Geometry: final body of the model. Coordinates: model frame, mm. A direction names the side the tool comes from. Round coordinates to 2 decimals unless told otherwise and drop trailing zeros. Loops run counter-clockwise (first coordinate to the right, second up) from the corner with the lowest first, then second, coordinate; pieces in that order, holes last. Notation, with made-up numbers: (18.25, 8.5) - (71.25, 8.5) arc R23 cw to (71.25, 47.5) - close; hole circle Ø1 at (-13, 6). An arc over 180 degrees is marked (long way). Write item = value, one per line. Start each with the question number.
Item 1: Section A-A (z = -12). Return loops of the section in (x, y).
Item 2: First-contact query: pin 1 (1 mm diameter, centred on x = 3.5, y = 3.5, fed in from +Z); pin 2 (4 mm diameter, centred on x = 0.5, y = -0.5, fed in from +Z); pin 3 (4 mm diameter, centred on y = 2.5, z = -5.5, fed in from -X). Flat tips, straight axial feed; report the tip coordinate or a pass-through.
Item 3: Line query: line 1 (Y direction, x = 0, z = -11.75); line 2 (Y direction, x = -3.5, z = -3.25). Output: solid intervals per line, ascending. Write a range as from..to.
Item 4: Draft query along Y for faces 3 (the conical face through (-2.24, 0.71, 5.54)), 4 (the cylindrical face through (-5.96, 1.88, -7.43)). Return one class per face: pulls with the +Y half, pulls with the -Y half, needs draft (parallel to the pull), parting line crosses it, or undercut.
Item 5: Access query for faces 1 (the cylindrical face through (-2.285, 3.584, -7.155)), 2 (the conical face through (-1.74, -3.345, 6.363)). Directions: +Z, -Z, +X, -X, +Y, -Y. A direction counts if a zero-diameter tool reaches every point of the face in a straight line with its end or side. Return the directions, or none.
from build123d import *

# Parameters (mm, degrees)
F2_R = 0.8


with BuildPart() as f1:
    # F0 (on Front) → F1 (revolve)
    with BuildSketch(Plane.XZ):
        Polygon((-4.25, 2.833334), (-1.375272, 6.924292), (-3.375272, 6.924292), (-6.25, 2.833334), (-6.25, -17.166666), (-4.25, -17.166666), align=None)
    revolve(axis=Axis((0, 0, -1.357143), (0, 0, -1)))

    # F2
    f2_edges = [f1.edges().sort_by_distance(p)[0] for p in [
        (1.375272, 0, 6.924292),
        (3.375272, 0, 6.924292),
        (6.25, 0, 2.833334),
        (4.25, 0, 2.833334),
        (-2.812636, 0, 4.878813),
    ]]
    fillet(f2_edges, radius=F2_R)


solid = f1.part
Taken from the geometry:
q1.outline = circle Ø12.5 at (0, 0); hole circle Ø8.5 at (0, 0)
q2.pin_1 = 5.4
q2.pin_2 = 6.9
q2.pin_3 = -6.23
q3.line_1 = -6.25..-4.25, 4.25..6.25
q3.line_2 = -5.18..-2.41, 2.41..5.18
q4.face_3 = undercut
q4.face_4 = parting line crosses it
q5.face_1 = -Z
q5.face_2 = +Z
